Work out the finished part from the listing and answer in its coordinate system (mm). A direction names the side the tool comes from. Coordinates: 2 decimals unless noted, no trailing zeros. Write each loop counter-clockwise with the first axis right and the second up, starting at its lowest first coordinate (ties: lowest second). Pieces come first, ordered by that corner, then holes. Notation, with made-up numbers: M 31,59.25 L 44,59.25 A12 cw 44,69.25 Z; hole C 20,33 d2. An arc over 180 degrees is marked long. Use CSV: the item, a comma, the result in double quotes.
from build123d import *

# Parameters (mm, degrees)
EXTRUDE_1_DEPTH          = 32
SHELL_1_T                = -10
SKETCH_2_R               = 36
CUT_EXTRUDE_1_DEPTH      = 3
SKETCH_3_R               = 36
CUT_EXTRUDE_2_DEPTH      = 3
FILLET_1_R               = 5
FILLET_2_R               = 10
PATTERN_CIRCULAR_1_COUNT = 6
PATTERN_CIRCULAR_2_COUNT = 6


with BuildPart() as part:
    # Эскиз1 → Бобышка-Вытянуть1 (new body, symmetric)
    with BuildSketch(Plane.XY):
        with BuildLine():
            Line((-38, 0), (-25, 0))
            ThreePointArc((-25, 0), (0, -25), (25, 0))
            Line((25, 0), (59, 0))
            ThreePointArc((59, 0), (84, -25), (109, 0))
            Line((109, 0), (162, 0))
            Line((162, 0), (162, -40))
            Line((162, -40), (122, -80))
            Line((122, -80), (2, -80))
            Line((2, -80), (-38, -40))
            Line((-38, -40), (-38, 0))
        make_face()
    extrude(amount=EXTRUDE_1_DEPTH, both=True)

    # Оболочка1
    shell_1_openings = [part.faces().sort_by_distance(p)[0] for p in [
        (-31.5, 0, 0),
        (0, -12.5, 0),
        (42, 0, 0),
        (84, -12.5, 0),
        (135.5, 0, 0),
    ]]
    offset(amount=SHELL_1_T, openings=shell_1_openings, kind=Kind.INTERSECTION)

    # Эскиз2 → Вырез-Вытянуть1 (cut)
    with BuildSketch(Plane.XY.offset(32)):
        Circle(SKETCH_2_R)
        with Locations((84, 0)):
            Circle(SKETCH_2_R)
    extrude(amount=-CUT_EXTRUDE_1_DEPTH, mode=Mode.SUBTRACT)

    # Эскиз3 → Вырез-Вытянуть2 (cut)
    with BuildSketch(Plane(origin=(0, 0, -32), x_dir=(-1, 0, 0), z_dir=(0, 0, -1))):
        Circle(SKETCH_3_R)
        with Locations((-84, 0)):
            Circle(SKETCH_3_R)
    extrude(amount=-CUT_EXTRUDE_2_DEPTH, mode=Mode.SUBTRACT)

    # Скругление1
    fillet_1_edges = [part.edges().sort_by_distance(p)[0] for p in [
        (-28, -17.928932188, -22),
        (-10.928932188, -52.928932188, -22),
        (-28, -35.857864376, 0),
        (62, -70, -22),
        (6.142135624, -70, 0),
        (134.928932188, -52.928932188, -22),
        (117.857864376, -70, 0),
        (152, -17.928932188, -22),
        (152, -35.857864376, 0),
        (-28, -17.928932188, 22),
        (-10.928932188, -52.928932188, 22),
        (62, -70, 22),
        (134.928932188, -52.928932188, 22),
        (152, -17.928932188, 22),
    ]]
    fillet(fillet_1_edges, radius=FILLET_1_R)

    # Скругление2
    fillet_2_edges = [part.edges().sort_by_distance(p)[0] for p in [
        (162, -40, 0),
        (122, -80, 0),
        (2, -80, 0),
        (-38, -40, 0),
    ]]
    fillet(fillet_2_edges, radius=FILLET_2_R)

    # Эскиз6 → Отверстие обработанное метчиком M61 (revolve, cut)
    with BuildSketch(Plane(origin=(0, -30, 29), x_dir=(0, -1, 0), z_dir=(1, 0, 0))):
        Polygon((0, 0), (0, 20.487130032), (2.475, 19), (2.475, 1), (3.475, 0), align=None)
    hole_wizard_m61 = revolve(axis=Axis((0, -30, 35.35), (0, 0, -1)), mode=Mode.SUBTRACT)

    # Эскиз8 → Отверстие обработанное метчиком M62 (revolve, cut)
    with BuildSketch(Plane(origin=(0, -30, -29), x_dir=(0, 1, 0), z_dir=(1, 0, 0))):
        Polygon((0, 0), (0, 20.487130032), (2.475, 19), (2.475, 1), (3.475, 0), align=None)
    hole_wizard_m62 = revolve(axis=Axis((0, -30, -35.35), (0, 0, 1)), mode=Mode.SUBTRACT)

    # Круговой массив1: Отверстие обработанное метчиком M61, Отверстие обработанное метчиком M62 ×6 about axis, 3 skipped
    pattern_circular_1_axis = Axis((0, 0, 0), (0, 0, 1))
    add([hole_wizard_m61.rotate(pattern_circular_1_axis, i * 360 / PATTERN_CIRCULAR_1_COUNT) for i in range(1, PATTERN_CIRCULAR_1_COUNT) if i not in (2, 3, 4)], mode=Mode.SUBTRACT)
    add([hole_wizard_m62.rotate(pattern_circular_1_axis, i * 360 / PATTERN_CIRCULAR_1_COUNT) for i in range(1, PATTERN_CIRCULAR_1_COUNT) if i not in (2, 3, 4)], mode=Mode.SUBTRACT)

    # Эскиз10 → Отверстие обработанное метчиком M63 (revolve, cut)
    with BuildSketch(Plane(origin=(84, -30, 29), x_dir=(0, -1, 0), z_dir=(1, 0, 0))):
        Polygon((0, 0), (0, 20.487130032), (2.475, 19), (2.475, 1), (3.475, 0), align=None)
    hole_wizard_m63 = revolve(axis=Axis((84, -30, 35.35), (0, 0, -1)), mode=Mode.SUBTRACT)

    # Эскиз12 → Отверстие обработанное метчиком M64 (revolve, cut)
    with BuildSketch(Plane(origin=(84, -30, -29), x_dir=(0, 1, 0), z_dir=(1, 0, 0))):
        Polygon((0, 0), (0, 20.487130032), (2.475, 19), (2.475, 1), (3.475, 0), align=None)
    hole_wizard_m64 = revolve(axis=Axis((84, -30, -35.35), (0, 0, 1)), mode=Mode.SUBTRACT)

    # Круговой массив2: Отверстие обработанное метчиком M63, Отверстие обработанное метчиком M64 ×6 about axis, 3 skipped
    pattern_circular_2_axis = Axis((84, 0, 0), (0, 0, -1))
    add([hole_wizard_m63.rotate(pattern_circular_2_axis, i * 360 / PATTERN_CIRCULAR_2_COUNT) for i in range(1, PATTERN_CIRCULAR_2_COUNT) if i not in (2, 3, 4)], mode=Mode.SUBTRACT)
    add([hole_wizard_m64.rotate(pattern_circular_2_axis, i * 360 / PATTERN_CIRCULAR_2_COUNT) for i in range(1, PATTERN_CIRCULAR_2_COUNT) if i not in (2, 3, 4)], mode=Mode.SUBTRACT)


solid = part.part
Item 1: Consider probe 1 along X at (y, z) = (-30, 24.1) (3 decimals); probe 2 along Z at (x, y) = (51, -8); probe 3 along Z at (x, y) = (128.5, -21). Determine where each line is inside the solid, lowest interval first.
Answer:
probe 1,"x = -38 to -2.475, 2.475 to 81.525, 86.475 to 162"
probe 2,"z = -29 to -22, 22 to 29"
probe 3,"z = -32 to -22, 22 to 32"
Item 2: The part is cut by section B-B (z = -25). Count the separate pieces of the cut face and the enclosed holes in it, then the cut area to 3 significant figures.
Answer:
separate pieces,"1"
enclosed holes,"6"
area,"12,300 mm2"
Item 3: A tool of negligible diameter and unlimited length cuts with its end or side. For faces 1 (the face through (55.603, -14.463, -25.042)), 2 (the face through (83.21, -35.99, 30.52)), 3 (the face through (-28.397, -15.537, 23.126)), 4 (the face through (63, -32, 22)), from which of +Z, -Z, +X, -X, +Y, -Y can it reach the whole face along a straight path? Write none if from no direction.
Answer:
face 1,"+Z, -Z"
face 2,"+Z, +Y"
face 3,"+Z"
face 4,"+Y"
Item 4: The part is cut by section A-A (z = 2.5). Write down the section's boundary in (x, y).
Answer:
outline,"M -38,-35.86 A10 ccw -35.07,-42.93 L -0.93,-77.07 A10 ccw 6.14,-80 L 117.86,-80 A10 ccw 124.93,-77.07 L 159.07,-42.93 A10 ccw 162,-35.86 L 162,0 L 152,0 L 152,-33.79 A5 cw 150.54,-37.32 L 119.32,-68.54 A5 cw 115.79,-70 L 8.21,-70 A5 cw 4.68,-68.54 L -26.54,-37.32 A5 cw -28,-33.79 L -28,0 L -38,0 Z"
Item 5: For a pull along Z with two mould halves and no side action, classify faces 5 (the face through (-27.63, -35.67, -0.24)), 6 (the face through (86.196, -28.858, -25.042)) as released by +Z, released by -Z, zero draft, split by the parting line, or undercut.
Answer:
face 5,"undercut"
face 6,"zero draft"
Item 6: Given pin 1 (6.5 mm diameter, centred on x = 0, y = -30, fed in from +Z) (3 decimals); pin 2 (4 mm diameter, centred on x = 109.98, y = -15, fed in from -Z); pin 3 (5.5 mm diameter, centred on x = 58.02, y = -15, fed in from +Z); pin 4 (8 mm diameter, centred on x = 25.98, y = -15, fed in from +Z), each flat-ended and moving along its own axis, determine where each tip first touches the part or whether it passes through.
Answer:
pin 1,"stops at z = 28.775"
pin 2,"passes through"
pin 3,"stops at z = 28.28"
pin 4,"stops at z = 29"
